Design review of the part built by this model. Coordinates are the model's own, in mm. A direction names the side the tool comes from. Round coordinates to 2 decimals unless told otherwise and drop trailing zeros. Order: outer loops, then holes, each group sorted by start corner. A loop starts at its lowest first (then second) coordinate and runs counter-clockwise, first axis right, second up.
from build123d import *

# Parameters (mm, degrees)
SKETCH_1_W                 = 8
SKETCH_1_H                 = 4
EXTRUDE_1_DEPTH            = 2
EXTRUDE_2_DEPTH            = 1.5
EXTRUDE_3_DEPTH            = 0.75
PATTERN_LINEAR_1_COUNT     = 2
PATTERN_LINEAR_1_PITCH     = 3
PATTERN_LINEAR_1_COL_COUNT = 2
PATTERN_LINEAR_1_COL_PITCH = 3


with BuildPart() as part:
    # 草图1 → 凸台-拉伸1 (new body)
    with BuildSketch(Plane(origin=(0, 0, 0), x_dir=(0, 0, -1), z_dir=(1, 0, 0))):
        Rectangle(SKETCH_1_W, SKETCH_1_H)
    extrude(amount=EXTRUDE_1_DEPTH)

    # 草图2 → 凸台-拉伸2 (add, symmetric)
    with BuildSketch(Plane.XY):
        Polygon((1, 2), (0, 4.215421364), (0, 3.49328806), (0.5, 2), align=None)
    extrude(amount=EXTRUDE_2_DEPTH, both=True)

    # 草图3 → 凸台-拉伸3 (add, symmetric)
    with BuildSketch(Plane.XY):
        Polygon((1, -2), (0, -4.472901544), (0, -3.77481073), (0.717703758, -2), align=None)
    extrude_3 = extrude(amount=EXTRUDE_3_DEPTH, both=True)

    # 阵列(线性)1: 凸台-拉伸3 ×2
    with Locations(*[(0, 0, i * PATTERN_LINEAR_1_PITCH) for i in range(1, PATTERN_LINEAR_1_COUNT)]):
        add(extrude_3)

    # 阵列(线性)1 col: 凸台-拉伸3 ×2
    with Locations(*[(0, 0, -i * PATTERN_LINEAR_1_COL_PITCH) for i in range(1, PATTERN_LINEAR_1_COL_COUNT)]):
        add(extrude_3)


solid = part.part
1) Take a section at A-A on x = 0.3. Give the boundary of the cut face in (y, z), plus the area to 3 significant figures.
Results:
outline: (-3.73, -3.75) - (-3.03, -3.75) - (-3.03, -2.25) - (-3.73, -2.25) - close; (-3.73, -0.75) - (-3.03, -0.75) - (-3.03, 0.75) - (-3.73, 0.75) - close; (-3.73, 2.25) - (-3.03, 2.25) - (-3.03, 3.75) - (-3.73, 3.75) - close; (-2, -4) - (2, -4) - (2, 4) - (-2, 4) - close; (2.6, -1.5) - (3.55, -1.5) - (3.55, 1.5) - (2.6, 1.5) - close
area: 38.0 mm2
2) Take a section at D-D on x = 1.6. Give the boundary of the cut face in (y, z).
Results:
outline: (-2, -4) - (2, -4) - (2, 4) - (-2, 4) - close
3) To check wall thickness, follow line 1 along Y through (x, z) = (1.5, -0.5); line 2 along Z through (x, y) = (0.4, 3.25); line 3 along Y through (x, z) = (0.5, 2.5). State the ranges of each line that lie inside material, in increasing order.
Results:
line 1: y = -2 to 2
line 2: z = -1.5 to 1.5
line 3: y = -3.24 to -2.54, -2 to 2
4) For faces 1 (the face through (0.247, 2.757, 0.021)), 2 (the face through (0.4, 2.9, -1.5)), 3 (the face through (1, 0, -4)), list the 3-axis set-ups (+Z, -Z, +X, -X, +Y, -Y) from which the entire face can be reached by the end or side of a thin tool; tool diameter is ignored.
Results:
face 1: +Z, -Z, -X
face 2: -Z, +X, -X, +Y
face 3: -Z, +X, -X, +Y, -Y
5) Take a section at C-C on y = -2.75. Give the boundary of the cut face in (x, z).
Results:
outline: (0.41, -3.75) - (0.7, -3.75) - (0.7, -2.25) - (0.41, -2.25) - close; (0.41, -0.75) - (0.7, -0.75) - (0.7, 0.75) - (0.41, 0.75) - close; (0.41, 2.25) - (0.7, 2.25) - (0.7, 3.75) - (0.41, 3.75) - close
6) Take a section at B-B on z = -0.25. Give the boundary of the cut face in (x, y), plus the area to 3 significant figures.
Results:
outline: (0, -4.47) - (1, -2) - (2, -2) - (2, 2) - (1, 2) - (0, 4.22) - (0, 3.49) - (0.5, 2) - (0, 2) - (0, -2) - (0.72, -2) - (0, -3.77) - close
area: 9.33 mm2
7) Clearance check with flat-ended pins moving along their axes: P1, Ø1.1, axis at x = 0.5, y = 3, coming from the -Z side; P2, Ø0.8, axis at x = 0.5, y = -3.5, coming from the -Z side; P3, Ø1.1, axis at x = 0.5, y = -3.5, coming from the +Z side. State where each tip first meets the part, or that it passes through.
Results:
P1: stops at z = -1.5
P2: stops at z = -3.75
P3: stops at z = 3.75
8) The part is to be moulded in two halves that separate along Y. For faces 4 (the face through (1.2, -2, 0.1)), 5 (the face through (0.507, -3.219, 3.01)), 6 (the face through (1, 0, 4)), say which applies: released by +Y, released by -Y, zero draft, split by the parting line, or undercut.
Results:
face 4: undercut
face 5: released by -Y
face 6: zero draft
